```python
from build123d import *

# Parameters (mm, degrees)
STOCK_HORN_DRIVE_FLANGE_START              = 41
STOCK_HORN_DRIVE_FLANGE_PROFILE_R          = 12
STOCK_HORN_DRIVE_FLANGE_PROFILE_R_2        = 4.05
STOCK_HORN_DRIVE_FLANGE_DEPTH              = 3
D_COUPLING_RING_START                      = 44
D_COUPLING_RING_PROFILE_R                  = 7
D_COUPLING_RING_PROFILE_R_2                = 4.05
D_COUPLING_RING_DEPTH                      = 4
D_KEY_LAND_START                           = 44
D_KEY_LAND_PROFILE_W                       = 2.9
D_KEY_LAND_PROFILE_H                       = 4.8
D_KEY_LAND_DEPTH                           = 4
STOCK_HORN_SCREWS_START                    = 39
STOCK_HORN_SCREWS_PROFILE_R                = 1.1
STOCK_HORN_SCREWS_DEPTH                    = 12.911688245
TWO_HORN_WASHER_CLEARANCES_START           = 44
TWO_HORN_WASHER_CLEARANCES_PROFILE_R       = 2.75
TWO_HORN_WASHER_CLEARANCES_DEPTH           = 4
YAW_POSITIVE_RETENTION_CROSSBOLT_START     = -10
YAW_POSITIVE_RETENTION_CROSSBOLT_PROFILE_R = 1.1
YAW_POSITIVE_RETENTION_CROSSBOLT_DEPTH     = 61.911688245
CROSSBOLT_FLAT_SEAT_CUT_12_START           = -12
CROSSBOLT_FLAT_SEAT_12_R                   = 2.75
CROSSBOLT_FLAT_SEAT_CUT_12_DEPTH           = 6
CROSSBOLT_FLAT_SEAT_CUT_6_START            = 6
CROSSBOLT_FLAT_SEAT_6_R                    = 2.75
CROSSBOLT_FLAT_SEAT_CUT_6_DEPTH            = 6


with BuildPart() as part:
    # Stock_horn_drive_flange_profile → Stock_horn_drive_flange (new body)
    with BuildSketch(Plane(origin=(0, 0, 0), x_dir=(1, 0, 0), z_dir=(0, 1, 0)).offset(STOCK_HORN_DRIVE_FLANGE_START)):
        with Locations(Location((0, 0, 0), (0, 0, 270))):
            Circle(STOCK_HORN_DRIVE_FLANGE_PROFILE_R)
        with Locations(Location((0, 0, 0), (0, 0, 270))):
            Circle(STOCK_HORN_DRIVE_FLANGE_PROFILE_R_2, mode=Mode.SUBTRACT)
    extrude(amount=STOCK_HORN_DRIVE_FLANGE_DEPTH)

    # D_coupling_ring_profile → D_coupling_ring (add)
    with BuildSketch(Plane(origin=(0, 0, 0), x_dir=(1, 0, 0), z_dir=(0, 1, 0)).offset(D_COUPLING_RING_START)):
        with Locations(Location((0, 0, 0), (0, 0, 270))):
            Circle(D_COUPLING_RING_PROFILE_R)
        with Locations(Location((0, 0, 0), (0, 0, 270))):
            Circle(D_COUPLING_RING_PROFILE_R_2, mode=Mode.SUBTRACT)
    extrude(amount=D_COUPLING_RING_DEPTH)

    # D_key_land_profile → D_key_land (add)
    with BuildSketch(Plane(origin=(0, 0, 0), x_dir=(1, 0, 0), z_dir=(0, 1, 0)).offset(D_KEY_LAND_START)):
        with Locations((4.55, 0)):
            Rectangle(D_KEY_LAND_PROFILE_W, D_KEY_LAND_PROFILE_H)
    extrude(amount=D_KEY_LAND_DEPTH)

    # Stock_horn_screws_profile → Stock_horn_screws (cut, through all)
    with BuildSketch(Plane(origin=(0, 0, 0), x_dir=(1, 0, 0), z_dir=(0, 1, 0)).offset(STOCK_HORN_SCREWS_START)):
        with Locations(Location((-8, 0, 0), (0, 0, 22.9239414))):
            Circle(STOCK_HORN_SCREWS_PROFILE_R)
        with Locations(Location((8, 0, 0), (0, 0, 157.0760586))):
            Circle(STOCK_HORN_SCREWS_PROFILE_R)
        with Locations(Location((0, -8, 0), (0, 0, 67.0760586))):
            Circle(STOCK_HORN_SCREWS_PROFILE_R)
        with Locations(Location((0, 8, 0), (0, 0, 292.9239414))):
            Circle(STOCK_HORN_SCREWS_PROFILE_R)
    extrude(amount=STOCK_HORN_SCREWS_DEPTH, mode=Mode.SUBTRACT)

    # Two_horn_washer_clearances_profile → Two_horn_washer_clearances (cut)
    with BuildSketch(Plane(origin=(0, 0, 0), x_dir=(1, 0, 0), z_dir=(0, 1, 0)).offset(TWO_HORN_WASHER_CLEARANCES_START)):
        with Locations((0, -8)):
            Circle(TWO_HORN_WASHER_CLEARANCES_PROFILE_R)
        with Locations((0, 8)):
            Circle(TWO_HORN_WASHER_CLEARANCES_PROFILE_R)
    extrude(amount=TWO_HORN_WASHER_CLEARANCES_DEPTH, mode=Mode.SUBTRACT)

    # Yaw_positive_retention_crossbolt_profile → Yaw_positive_retention_crossbolt (cut, through all)
    with BuildSketch(Plane(origin=(0, 0, 0), x_dir=(0, 0, -1), z_dir=(1, 0, 0)).offset(YAW_POSITIVE_RETENTION_CROSSBOLT_START)):
        with Locations(Location((0, 45.5, 0), (0, 0, 180))):
            Circle(YAW_POSITIVE_RETENTION_CROSSBOLT_PROFILE_R)
    extrude(amount=YAW_POSITIVE_RETENTION_CROSSBOLT_DEPTH, mode=Mode.SUBTRACT)

    # Crossbolt_flat_seat_-12 → Crossbolt_flat_seat_cut_-12 (cut)
    with BuildSketch(Plane(origin=(0, 0, 0), x_dir=(0, 0, -1), z_dir=(1, 0, 0)).offset(CROSSBOLT_FLAT_SEAT_CUT_12_START)):
        with Locations((0, 45.5)):
            Circle(CROSSBOLT_FLAT_SEAT_12_R)
    extrude(amount=CROSSBOLT_FLAT_SEAT_CUT_12_DEPTH, mode=Mode.SUBTRACT)

    # Crossbolt_flat_seat_6 → Crossbolt_flat_seat_cut_6 (cut)
    with BuildSketch(Plane(origin=(0, 0, 0), x_dir=(0, 0, -1), z_dir=(1, 0, 0)).offset(CROSSBOLT_FLAT_SEAT_CUT_6_START)):
        with Locations((0, 45.5)):
            Circle(CROSSBOLT_FLAT_SEAT_6_R)
    extrude(amount=CROSSBOLT_FLAT_SEAT_CUT_6_DEPTH, mode=Mode.SUBTRACT)


solid = part.part
```
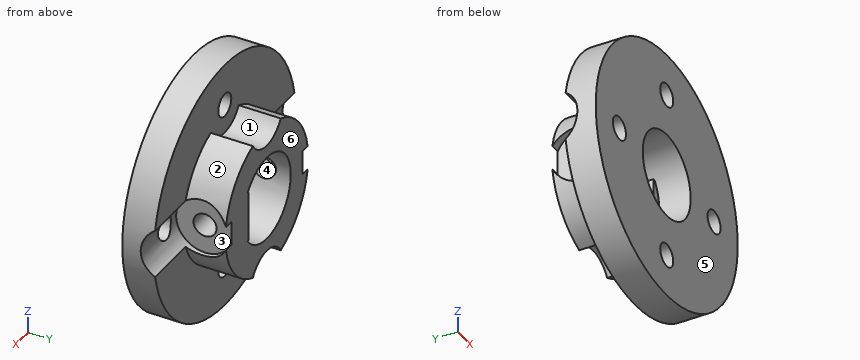
Geometry check sheet. Reference: the model listing, model coordinates, mm. Face numbers are marked on the shaded views. A direction names the side the tool comes from. Coordinates: 2 decimals unless noted, no trailing zeros. Order: outer loops, then holes, each group sorted by start corner. A loop starts at its lowest first (then second) coordinate and runs counter-clockwise, first axis right, second up. Notation, with made-up numbers: (71.25, 88) - (121.25, 88) arc R18 ccw to (121.25, 94) - close; hole circle Ø3 at (-33, -36). An arc over 180 degrees is marked (long way). Answer in a Markdown table with one row per item. Add a question column.
1. Section check A-A (x = 0). Enter the section's corners in (y, z).
2. Draft check along Y on the marked faces 4, 5 and 6. Enter one of: +Y half, -Y half, draft (parallel to the pull), parting line (faces both ways), or undercut.
3. Section check D-D (z = 8). Enter the section's corners in (x, y).
4. Material ranges on L1, parallel to Z at x = 0, y = 41.8; L2, parallel to Y at x = 4.2, z = 0; L3, parallel to X at y = 47.25, z = 0.25, recorded low to high. Write a range as [from, to].
5. Section check B-B (z = 0). Give the number of separate pieces and of enclosed holes in the cut face, plus the area to 3 significant figures.
6. Access from +Z, -Z, +X, -X, +Y, -Y to the whole of each face (thin tool, end or side, straight path). Record for the marked faces 1, 2 and 3.
7. Section check C-C (y = 45.5). Enter the section's corners in (x, z).
8. Gauge pin test, flat ends, axial feed: pin 1 Ø1.5 at (x, y) = (-1, 42.5) entering from +Z; pin 2 Ø2.5 at (y, z) = (45.5, 0) entering from -X; pin 3 Ø4 at (y, z) = (44.5, 8) entering from -X. Record the tip position at first contact, or that the pin passes through.
Data:
| question | item | result |
|---|---|---|
| 1 | outline | (41, -12) - (44, -12) - (44, -9.1) - (41, -9.1) - close; (41, -6.9) - (44, -6.9) - (44, -5.25) - (48, -5.25) - (48, -4.05) - (41, -4.05) - close; (41, 4.05) - (48, 4.05) - (48, 5.25) - (44, 5.25) - (44, 6.9) - (41, 6.9) - close; (41, 9.1) - (44, 9.1) - (44, 12) - (41, 12) - close |
| 2 | face 4 | undercut |
| 2 | face 5 | -Y half |
| 2 | face 6 | +Y half |
| 3 | outline | (-8.94, 41) - (-1.1, 41) - (-1.1, 44) - (-8.94, 44) - close; (1.1, 41) - (8.94, 41) - (8.94, 44) - (1.1, 44) - close |
| 4 | L1 | z = [-12, -9.1], [-6.9, -4.05], [4.05, 6.9], [9.1, 12] |
| 4 | L2 | y = [41, 44.4], [46.6, 48] |
| 4 | L3 | x = [-6, -4.04], [3.1, 6] |
| 5 | separate pieces | 6 |
| 5 | enclosed holes | 0 |
| 5 | area | 33.7 mm² |
| 6 | face 1 | +Z, +Y |
| 6 | face 2 | +Z, +X, +Y |
| 6 | face 3 | +X |
| 7 | outline | (-6.44, -2.75) arc R7 ccw to (-2.36, -6.59) arc R2.75 cw to (2.36, -6.59) arc R7 ccw to (6.44, -2.75) - (6, -2.75) - (6, -1.1) - (3.1, -1.1) - (3.1, -2.4) - (3.26, -2.4) arc R4.05 cw to (-3.9, -1.1) - (-6, -1.1) - (-6, -2.75) - close; (-6.44, 2.75) - (-6, 2.75) - (-6, 1.1) - (-3.9, 1.1) arc R4.05 cw to (3.26, 2.4) - (3.1, 2.4) - (3.1, 1.1) - (6, 1.1) - (6, 2.75) - (6.44, 2.75) arc R7 ccw to (2.36, 6.59) arc R2.75 cw to (-2.36, 6.59) arc R7 ccw to start |
| 8 | pin 1 | stops at z = 12 |
| 8 | pin 2 | stops at x = -6 |
| 8 | pin 3 | stops at x = -10.36 |
